```python
from build123d import *

# Parameters (mm, degrees)
SKETCH_W        = 252.15
SKETCH_H        = 80.7
SKETCH_R        = 1.225
SKETCH_R_2      = 1.975
PAD_DEPTH       = 18.6
SKETCH001_W     = 248.15
SKETCH001_H     = 76.7
POCKET_DEPTH    = 16.6
FILLET_R        = 2.3813
FILLET001_R     = 3.57195
SKETCH002_W     = 14
SKETCH002_H     = 2
POCKET001_DEPTH = 16.6
SKETCH003_W     = 131.259314
SKETCH003_H     = 131.259314
POCKET002_DEPTH = 20


with BuildPart() as part:
    # Sketch → Pad (new body)
    with BuildSketch(Plane.XY):
        Rectangle(SKETCH_W, SKETCH_H)
        with Locations((-104.775, 19.05)):
            Circle(SKETCH_R, mode=Mode.SUBTRACT)
        with Locations((-28.575, 19.05)):
            Circle(SKETCH_R, mode=Mode.SUBTRACT)
        with Locations((-6.3189, -19.05)):
            Circle(SKETCH_R_2, mode=Mode.SUBTRACT)
        with Locations((-104.775, -19.05)):
            Circle(SKETCH_R, mode=Mode.SUBTRACT)
        with Locations((-28.575, -19.05)):
            Circle(SKETCH_R, mode=Mode.SUBTRACT)
        with Locations((6.3189, -19.05)):
            Circle(SKETCH_R_2, mode=Mode.SUBTRACT)
        with Locations((28.575, -19.05)):
            Circle(SKETCH_R, mode=Mode.SUBTRACT)
        with Locations((28.575, 19.05)):
            Circle(SKETCH_R, mode=Mode.SUBTRACT)
        with Locations((104.775, 19.05)):
            Circle(SKETCH_R, mode=Mode.SUBTRACT)
        with Locations((104.775, -19.05)):
            Circle(SKETCH_R, mode=Mode.SUBTRACT)
    extrude(amount=PAD_DEPTH)

    # Sketch001 (on Face16 of Pad) → Pocket (cut)
    with BuildSketch(Plane.XY.offset(18.6)):
        Rectangle(SKETCH001_W, SKETCH001_H)
    extrude(amount=-POCKET_DEPTH, mode=Mode.SUBTRACT)

    # Fillet
    fillet_edges = [part.edges().sort_by_distance(p)[0] for p in [
        (-124.075, 38.35, 10.3),
        (-124.075, -38.35, 10.3),
        (124.075, 38.35, 10.3),
        (124.075, -38.35, 10.3),
    ]]
    fillet(fillet_edges, radius=FILLET_R)

    # Fillet001
    fillet001_edges = [part.edges().sort_by_distance(p)[0] for p in [
        (-126.075, 40.35, 9.3),
        (-126.075, -40.35, 9.3),
        (126.075, -40.35, 9.3),
        (126.075, 40.35, 9.3),
    ]]
    fillet(fillet001_edges, radius=FILLET001_R)

    # Sketch002 (on Face1 of Fillet001) → Pocket001 (cut)
    with BuildSketch(Plane.XY.offset(18.6)):
        with Locations((0, 39.35)):
            Rectangle(SKETCH002_W, SKETCH002_H)
    extrude(amount=-POCKET001_DEPTH, mode=Mode.SUBTRACT)

    # Sketch003 (on Face1 of Pocket001) → Pocket002 (cut)
    with BuildSketch(Plane.XY.offset(18.6)):
        with Locations((65.629657, 0)):
            Rectangle(SKETCH003_W, SKETCH003_H)
    extrude(amount=-POCKET002_DEPTH, mode=Mode.SUBTRACT)


solid = part.part
```
Can you work these out from the model? Positions are in its coordinate system, mm. A direction names the side the tool comes from. Coordinates: 2 decimals unless noted, no trailing zeros. Order: outer loops, then holes, each group sorted by start corner. A loop starts at its lowest first (then second) coordinate and runs counter-clockwise, first axis right, second up. Notation, with made-up numbers: (-40, 9.5) - (5, 9.5) arc R10 ccw to (5, 18.5) - close; hole circle Ø2 at (-2, 12.25). An arc over 180 degrees is marked (long way). Answer in a Markdown table with one row per item.
1. Suppose I cut it at B-B (y = -19.05). Please give me the cut outline in (x, z) (3 decimals).
Reply:
| item | result |
|---|---|
| outline | (-126.075, 0) - (-106, 0) - (-106, 2) - (-124.075, 2) - (-124.075, 18.6) - (-126.075, 18.6) - close; (-103.55, 0) - (-29.8, 0) - (-29.8, 2) - (-103.55, 2) - close; (-27.35, 0) - (-8.294, 0) - (-8.294, 2) - (-27.35, 2) - close; (-4.344, 0) - (0, 0) - (0, 2) - (-4.344, 2) - close |
2. Suppose I cut it at D-D (x = -79). Please give me the cut outline in (y, z).
Reply:
| item | result |
|---|---|
| outline | (-40.35, 0) - (40.35, 0) - (40.35, 18.6) - (38.35, 18.6) - (38.35, 2) - (-38.35, 2) - (-38.35, 18.6) - (-40.35, 18.6) - close |
3. For faces 1 (the flat face through (-62, -40.35, 9)), 2 (the cylindrical face through (-123.36, 37.67, 10.18)), which set-ups out of +Z, -Z, +X, -X, +Y, -Y let a thin tool reach every point of the face, with its end or its side?
Reply:
| item | result |
|---|---|
| face 1 | +Z, -Z, +X, -X, -Y |
| face 2 | +Z, +X |
4. Suppose I cut it at A-A (y = 19.05). Please give me the cut outline in (x, z) (3 decimals).
Reply:
| item | result |
|---|---|
| outline | (-126.075, 0) - (-106, 0) - (-106, 2) - (-124.075, 2) - (-124.075, 18.6) - (-126.075, 18.6) - close; (-103.55, 0) - (-29.8, 0) - (-29.8, 2) - (-103.55, 2) - close; (-27.35, 0) - (0, 0) - (0, 2) - (-27.35, 2) - close |
5. For pin 1 (2 mm diameter, centred on x = -28.575, y = -19.05, fed in from -Z); pin 2 (2 mm diameter, centred on x = -15.5, y = -6, fed in from +Z); pin 3 (1 mm diameter, centred on y = 39, z = 9, fed in from +X); pin 4 (8.5 mm diameter, centred on y = 6.5, z = 12, fed in from +X) (3 decimals), each with a flat end and sliding along its axis, tell me the tip position at first contact or that it passes through.
Reply:
| item | result |
|---|---|
| pin 1 | passes through |
| pin 2 | stops at z = 2 |
| pin 3 | stops at x = -7 |
| pin 4 | stops at x = -124.075 |
6. If we mould it in two halves opening along X, with no side actions, what happens to faces 3 (the cylindrical face through (-29.547, -19.795, 0.986)), 4 (the flat face through (-126.075, -1, 9)), 5 (the cylindrical face through (-123.36, -37.67, 10.18))? For each: pulls with the +X half, pulls with the -X half, needs draft (parallel to the pull), parting line crosses it, or undercut.
Reply:
| item | result |
|---|---|
| face 3 | undercut |
| face 4 | pulls with the -X half |
| face 5 | pulls with the +X half |
7. Suppose I cut it at C-C (z = 4.25). Please give me the cut outline in (x, y) (3 decimals), and give its area (3 significant figures).
Reply:
| item | result |
|---|---|
| outline | (-126.075, -36.778) arc R3.572 ccw to (-122.503, -40.35) - (0, -40.35) - (0, -38.35) - (-121.694, -38.35) arc R2.381 cw to (-124.075, -35.969) - (-124.075, 35.969) arc R2.381 cw to (-121.694, 38.35) - (-7, 38.35) - (-7, 40.35) - (-122.503, 40.35) arc R3.572 ccw to (-126.075, 36.778) - close |
| area | 641 mm^2 |
8. If I drill on line 1 along X through (y, z) = (19.05, 1.5) (3 decimals); line 2 along X through (y, z) = (-19.05, 1.1) (3 decimals); line 3 along Y through (x, z) = (-93, 15.5), over which ranges is the centre line in solid material (lowest first)?
Reply:
| item | result |
|---|---|
| line 1 | x = -126.075 to -106, -103.55 to -29.8, -27.35 to 0 |
| line 2 | x = -126.075 to -106, -103.55 to -29.8, -27.35 to -8.294, -4.344 to 0 |
| line 3 | y = -40.35 to -38.35, 38.35 to 40.35 |
